Build history of the part. All positions in model axes, mm. A direction names the side the tool comes from. Round coordinates to 2 decimals unless told otherwise and drop trailing zeros. Loops run counter-clockwise (first coordinate to the right, second up) from the corner with the lowest first, then second, coordinate; pieces in that order, holes last. Notation, with made-up numbers: M 17,-38 L 67,-38 A19 ccw 67,-2 Z; hole C 17.25,-37.5 d8. An arc over 180 degrees is marked long. Use one line per item in the form item = value. Start each with the question number.
```python
from build123d import *

# Parameters (mm, degrees)
EXTRUDE_1_DEPTH     = 3
FILLET_1_R          = 0.5
FILLET_2_R          = 1.25
SKETCH_3_R          = 1.6
CUT_EXTRUDE_2_DEPTH = 16.008331163
SKETCH_4_R          = 2.05
CUT_EXTRUDE_4_DEPTH = 4
CUT_EXTRUDE_5_DEPTH = 16.008331163


with BuildPart() as part:
    # ｽｹｯﾁ1 → ﾎﾞｽ - 押し出し1 (new, symmetric)
    with BuildSketch(Plane.XY):
        Polygon((1.5, 14), (-1.5, 14), (-1.5, 5), (-3, 5), (-3, 0), (3, 0), (3, 5), (1.5, 5), align=None)
    extrude(amount=EXTRUDE_1_DEPTH, both=True)

    # ﾌｨﾚｯﾄ1
    fillet_1_edges = [part.edges().sort_by_distance(p)[0] for p in [
        (1.5, 5, 0),
        (3, 0, 0),
        (-3, 0, 0),
        (-1.5, 5, 0),
    ]]
    fillet(fillet_1_edges, radius=FILLET_1_R)

    # ﾌｨﾚｯﾄ2
    fillet_2_edges = [part.edges().sort_by_distance(p)[0] for p in [
        (3, 5, 0),
        (-3, 5, 0),
    ]]
    fillet(fillet_2_edges, radius=FILLET_2_R)

    # ｽｹｯﾁ3 → ｶｯﾄ - 押し出し2 (cut, through all)
    with BuildSketch(Plane.ZY.offset(1.5)):
        with Locations(Location((0, 11, 0), (0, 0, 270))):
            Circle(SKETCH_3_R)
    extrude(amount=-CUT_EXTRUDE_2_DEPTH, mode=Mode.SUBTRACT)

    # ｽｹｯﾁ4 → ｶｯﾄ - 押し出し4 (cut)
    with BuildSketch(Plane.XZ):
        with Locations(Location((0, 0, 0), (0, 0, 270))):
            Circle(SKETCH_4_R)
    extrude(amount=-CUT_EXTRUDE_4_DEPTH, mode=Mode.SUBTRACT)

    # ｽｹｯﾁ5 → ｶｯﾄ - 押し出し5 (cut, through all)
    with BuildSketch(Plane.ZY.offset(1.5)):
        with BuildLine():
            Line((-3, 14), (-3, 11))
            ThreePointArc((-3, 11), (-2.121320344, 13.121320344), (0, 14))
            Line((0, 14), (-3, 14))
        make_face()
        with BuildLine():
            Line((3, 14), (0, 14))
            ThreePointArc((0, 14), (2.121320344, 13.121320344), (3, 11))
            Line((3, 11), (3, 14))
        make_face()
    extrude(amount=-CUT_EXTRUDE_5_DEPTH, mode=Mode.SUBTRACT)


solid = part.part
```
Q1. Saw through at A-A (x = 0). Give the cut face in (y, z), and give its area (3 significant figures).
Q2. Saw through at C-C (y = 12). Give the cut face in (x, z), and give its area (3 significant figures).
Q3. Wall check: probe 1 along Z at (x, y) = (-0.05, 11); probe 2 along X at (y, z) = (3.15, 0); probe 3 along X at (y, z) = (9.25, 2.5). Give the ranges that are in metal, low to high.
Q4. Saw through at D-D (x = -1.75). Give the cut face in (y, z).
Q5. Pull direction Z, two halves, no side cores. Call faces 4 (the face through (0, 4, -3)), 5 (the face through (2.033, 1.972, 0.267)), 6 (the face through (3, 2, 0)): pulls with the +Z half, pulls with the -Z half, needs draft (parallel to the pull), parting line crosses it, or undercut.
Q6. Drop flat-ended pins along their axis: P1, Ø2.5, axis at x = 0, z = 0, coming from the -Y side; P2, Ø1.8, axis at y = 9.5, z = 0.5, coming from the +X side; P3, Ø3.5, axis at y = 11, z = 0, coming from the -X side. Give the stop position or say it passes through.
Q7. Tool access for faces 1 (the face through (0, 4, 0)), 2 (the face through (1.5, 9, 0)), 3 (the face through (-1.5, 9, 0)): list every direction of +Z, -Z, +X, -X, +Y, -Y with a clear straight run to the whole face (end or side of a thin tool).
Q8. Saw through at B-B (y = 1). Give the cut face in (x, z).
Filled in:
q1.outline = M 0,-3 L 11,-3 A3 ccw 11,3 L 0,3 L 0,2.05 L 4,2.05 L 4,-2.05 L 0,-2.05 Z; hole C 11,0 d3.2
q1.area = 55.7 mm²
q2.outline = M -1.5,-2.83 L 1.5,-2.83 L 1.5,-1.25 L -1.5,-1.25 Z; M -1.5,1.25 L 1.5,1.25 L 1.5,2.83 L -1.5,2.83 Z
q2.area = 9.48 mm²
q3.probe_1 = -3 to -1.6, 1.6 to 3
q3.probe_2 = -3 to -2.05, 2.05 to 3
q3.probe_3 = -1.5 to 1.5
q4.outline = M 0,-3 L 5.07,-3 L 5.07,3 L 0,3 L 0,1.07 L 4,1.07 L 4,-1.07 L 0,-1.07 Z
q5.face_4 = pulls with the -Z half
q5.face_5 = undercut
q5.face_6 = needs draft
q6.P1 = 4
q6.P2 = 1.5
q6.P3 = -1.5
q7.face_1 = -Y
q7.face_2 = +Z, -Z, +X, +Y
q7.face_3 = +Z, -Z, -X, +Y
q8.outline = M -3,-3 L 3,-3 L 3,3 L -3,3 Z; hole C 0,0 d4.1
